Verification items for this drawing (mm, ordinates from the low corner). A direction names the side the tool comes from. Round coordinates to 2 decimals unless told otherwise and drop trailing zeros. Write each loop counter-clockwise with the first axis right and the second up, starting at its lowest first coordinate (ties: lowest second). Pieces come first, ordered by that corner, then holes.
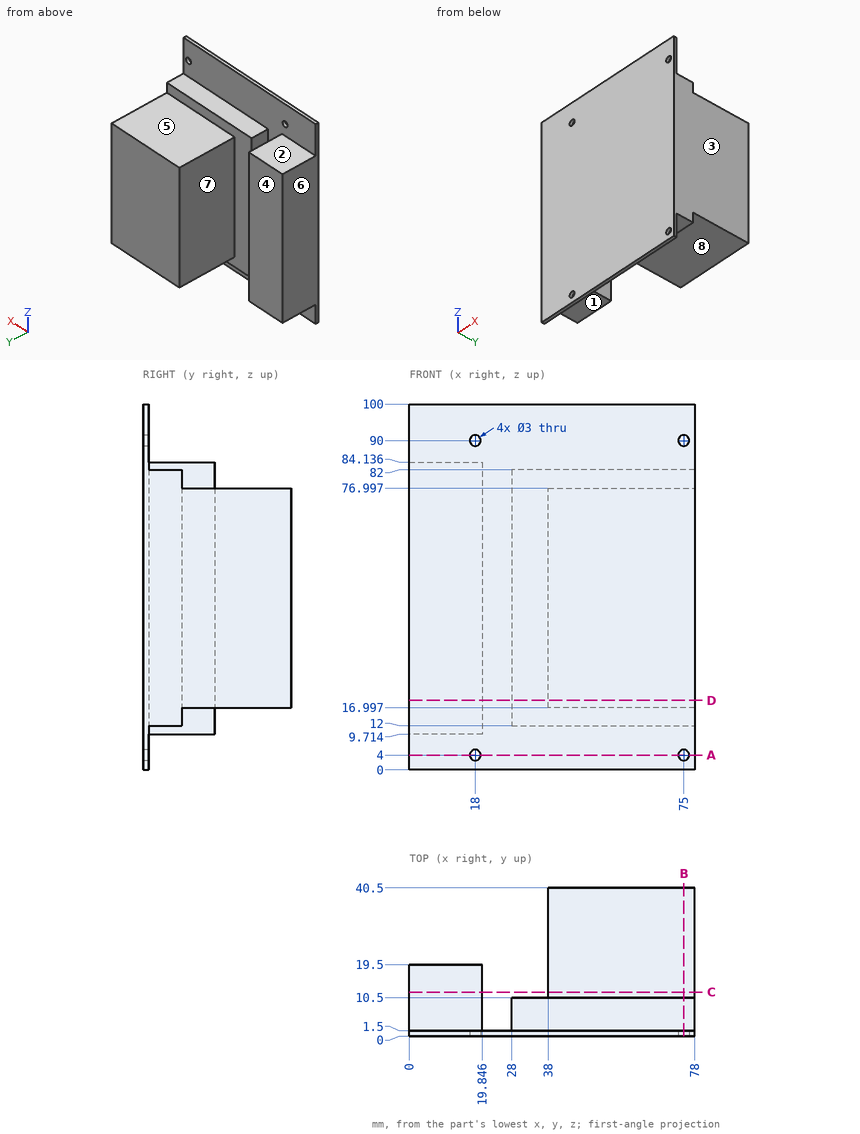
1. Depth check by flat-ended pin: pin 1 Ø4.5 at (x, y) = (58, 6) entering from -Z; pin 2 Ø4 at (x, z) = (29.5, 56.5) entering from +Y; pin 3 Ø2 at (x, z) = (13, 80) entering from +Y. Enter the tip coordinate at first touch or a pass-through.
2. Access from +Z, -Z, +X, -X, +Y, -Y to the whole of each face (thin tool, end or side, straight path). Record for the marked faces 1, 2, 3, 4 and 5.
3. Section check B-B (x = 75). Record the cut outline in (y, z).
4. Section check C-C (y = 12). Record the cut outline in (x, z).
5. Release check for a two-part mould opening along X. For the marked faces 6, 7 and 8 record: +X half, -X half, draft (parallel to the pull), parting line (faces both ways), or undercut.
6. Section check A-A (z = 4). Record the cut outline in (x, y), plus the area to 3 significant figures.
7. Section check D-D (z = 19). Record the cut outline in (x, y), plus the area to 3 significant figures.
8. Scan lines: line 1 along X through (y, z) = (1, 4); line 2 along Z through (x, y) = (18, 1); line 3 along X through (y, z) = (7, 50). Record each from-to range of solid material in increasing order.
Results below:
1. pin 1: stops at z = 12
1. pin 2: stops at y = 10.5
1. pin 3: stops at y = 19.5
2. face 1: -Z, +X, -X, +Y
2. face 2: +Z, +X, -X, +Y
2. face 3: +Z, -Z, +X, +Y, -Y
2. face 4: +Z, -Z, -X, +Y
2. face 5: +Z, +X, +Y
3. outline: (0, 0) - (1.5, 0) - (1.5, 2.5) - (0, 2.5) - close; (0, 5.5) - (1.5, 5.5) - (1.5, 12) - (10.5, 12) - (10.5, 17) - (40.5, 17) - (40.5, 77) - (10.5, 77) - (10.5, 82) - (1.5, 82) - (1.5, 88.5) - (0, 88.5) - close; (0, 91.5) - (1.5, 91.5) - (1.5, 100) - (0, 100) - close
4. outline: (0, 9.71) - (19.85, 9.71) - (19.85, 84.14) - (0, 84.14) - close; (38, 17) - (78, 17) - (78, 77) - (38, 77) - close
5. face 6: -X half
5. face 7: undercut
5. face 8: draft
6. outline: (0, 0) - (16.5, 0) - (16.5, 1.5) - (0, 1.5) - close; (19.5, 0) - (73.5, 0) - (73.5, 1.5) - (19.5, 1.5) - close; (76.5, 0) - (78, 0) - (78, 1.5) - (76.5, 1.5) - close
6. area: 108 mm2
7. outline: (0, 0) - (78, 0) - (78, 40.5) - (38, 40.5) - (38, 10.5) - (28, 10.5) - (28, 1.5) - (19.85, 1.5) - (19.85, 19.5) - (0, 19.5) - close
7. area: 2,120 mm2
8. line 1: x = 0 to 16.5, 19.5 to 73.5, 76.5 to 78
8. line 2: z = 0 to 2.5, 5.5 to 88.5, 91.5 to 100
8. line 3: x = 0 to 19.85, 28 to 78
